Work out the finished part from the listing and answer in its coordinate system (mm). A direction names the side the tool comes from. Coordinates: 2 decimals unless noted, no trailing zeros. Order: outer loops, then holes, each group sorted by start corner. A loop starts at its lowest first (then second) coordinate and runs counter-clockwise, first axis right, second up.
1. Find the intervals of material crossed by probe 1 along Y at (x, z) = (-4.6, -1.75); probe 2 along X at (y, z) = (2.45, -4.25); probe 3 along X at (y, z) = (2.65, -5.5), in increasing order.
2. The part is cut by section B-B, the plane z = -5.5. Give the vertices of the cut face in (x, y), then the cut area to 3 significant figures.
3. A tool of negligible diameter and unlimited length cuts with its end or side. For faces 1 (the flat face through (-3, 2, -1)), 2 (the flat face through (-3, 2, -6)), 3 (the flat face through (-2.7, 0, -3.4)), from which of +Z, -Z, +X, -X, +Y, -Y can it reach the whole face along a straight path? Write none if from no direction.
4. The part is cut by section A-A, the plane y = 2.2. Give the vertices of the cut face in (x, z).
5. Flat-ended cylindrical pins translate along their axes: pin 1 Ø1 at (y, z) = (1, -2.5) entering from +X; pin 2 Ø1.8 at (x, z) = (-3, -4) entering from +Y. Find the tip coordinate at first contact, or state that the pin passes through.
6. The part is cut by section D-D, the plane y = 1.9. Give the vertices of the cut face in (x, z).
7. Determine the mould class of faces 4 (the flat face through (-4.6, 2.8, -3.4)), 5 (the flat face through (-3, 2.1, -3)), 6 (the cylindrical face through (-2.31, 1.75, -1.36)) for opening direction Z: +Z half, -Z half, draft (parallel to the pull), parting line (faces both ways), or undercut.
8. The part is cut by section C-C, the plane y = 2.65. Give the vertices of the cut face in (x, z), then the cut area to 3 significant figures.
Autodesk Inventor part; units mm, degrees
ref_plane "YZ Plane" through (0, 0, 0) normal (1, 0, 0) x (0, 1, 0)
ref_plane "XZ Plane" through (0, 0, 0) normal (0, 1, 0) x (-1, 0, 0)
ref_plane "XY Plane" through (0, 0, 0) normal (0, 0, 1) x (1, 0, 0)
sketch "Skizze1" plane through (0, 0, 0) normal (0, 1, 0) x (-1, 0, 0)
  circle A0 centre (2.7514, -3.3638) radius 2.05
  point P0 (0, 0)
  dimension "d0" = 4.1
extrude "Extrusion1" add sketch "Skizze1" along normal blind 2
fillet "Rundung1" radius 1.5 1 edges at (-0.7014, 0, -3.3638)
sketch "Skizze9" plane through (-2.7514, 2, -3.3638) normal (0, 1, 0) x (1, 0, 0)
  point P0 (2.7514, -3.3638)
sketch "Skizze10" plane through (-2.7514, 2, -3.3638) normal (0, 1, 0) x (1, 0, 0)
  line L0 (0, 0) -> (2.05, 0)
  line L1 (2.05, 0) -> (2.05, 3.3)
  line L2 (2.05, 3.3) -> (0, 3.3)
  line L3 (0, 3.3) -> (0, 0)
  line L4 (2.05, 3.3) -> (-2.05, 3.3)
  line L5 (-2.05, 3.3) -> (-2.05, -3.3)
  line L6 (-2.05, -3.3) -> (2.05, -3.3)
  line L7 (2.05, -3.3) -> (2.05, 3.3)
  point P0 (2.7514, -3.3638)
  point P1 (0, 3.3)
  dimension "d27" = 3.3
  dimension "d28" = 6.6
extrude "Extrusion9" add sketch "Skizze10" along normal blind 0.8
sketch "Skizze12" plane through (-2.7514, 2.8, -3.3638) normal (0, 1, 0) x (1, 0, 0)
  line L0 (-0.0005, -0.0013) -> (-0.8005, -0.0013)
  line L1 (-0.8005, -0.0013) -> (-0.8005, 1.7987)
  line L2 (-0.8005, 1.7987) -> (-0.0005, 1.7987)
  line L3 (-0.0005, 1.7987) -> (-0.0005, -0.0013)
  line L4 (-0.8005, 1.7987) -> (0.7995, 1.7987)
  line L5 (0.7995, 1.7987) -> (0.7995, -1.8013)
  line L6 (0.7995, -1.8013) -> (-0.8005, -1.8013)
  line L7 (-0.8005, -1.8013) -> (-0.8005, 1.7987)
  point P0 (2.7514, -3.3638)
  dimension "d35" = 0.8
  dimension "d36" = 1.8
  dimension "d37" = 1.6
  dimension "d38" = 3.6
extrude "Extrusion10" cut sketch "Skizze12" against normal blind 0.7
chamfer "Fase1" distance 0.7 angle 45 4 edges at (-1.9519, 2.8, -3.3625) (-3.5519, 2.8, -3.3625) (-2.7519, 2.8, -5.1625) (-2.7519, 2.8, -1.5625)
properties part number "button" material "Gummi, Silikon"
Geometry says:
1. probe 1: y = 2 to 2.8
1. probe 2: x = -4.8 to -3.9, -1.6 to -0.7
1. probe 3: x = -4.8 to -4.1, -1.4 to -0.7
2. outline: (-4.8, 2) - (-0.7, 2) - (-0.7, 2.8) - (-1.25, 2.8) - (-1.61, 2.44) - (-3.89, 2.44) - (-4.25, 2.8) - (-4.8, 2.8) - close
2. area: 2.33 mm2
3. face 1: +Z, -Y
3. face 2: -Z, -Y
3. face 3: +Z, -Z, +X, -X, -Y
4. outline: (-4.8, -6.66) - (-0.7, -6.66) - (-0.7, -0.06) - (-4.8, -0.06) - close; hole (-3.65, -5.26) - (-1.85, -5.26) - (-1.85, -1.46) - (-3.65, -1.46) - close
5. pin 1: stops at x = -0.77
5. pin 2: stops at y = 2.45
6. outline: circle Ø4.1 at (-2.75, -3.36)
7. face 4: draft
7. face 5: undercut
7. face 6: parting line
8. outline: (-4.8, -6.66) - (-0.7, -6.66) - (-0.7, -0.06) - (-4.8, -0.06) - close; hole (-4.1, -5.71) - (-1.4, -5.71) - (-1.4, -1.01) - (-4.1, -1.01) - close
8. area: 14.4 mm2
